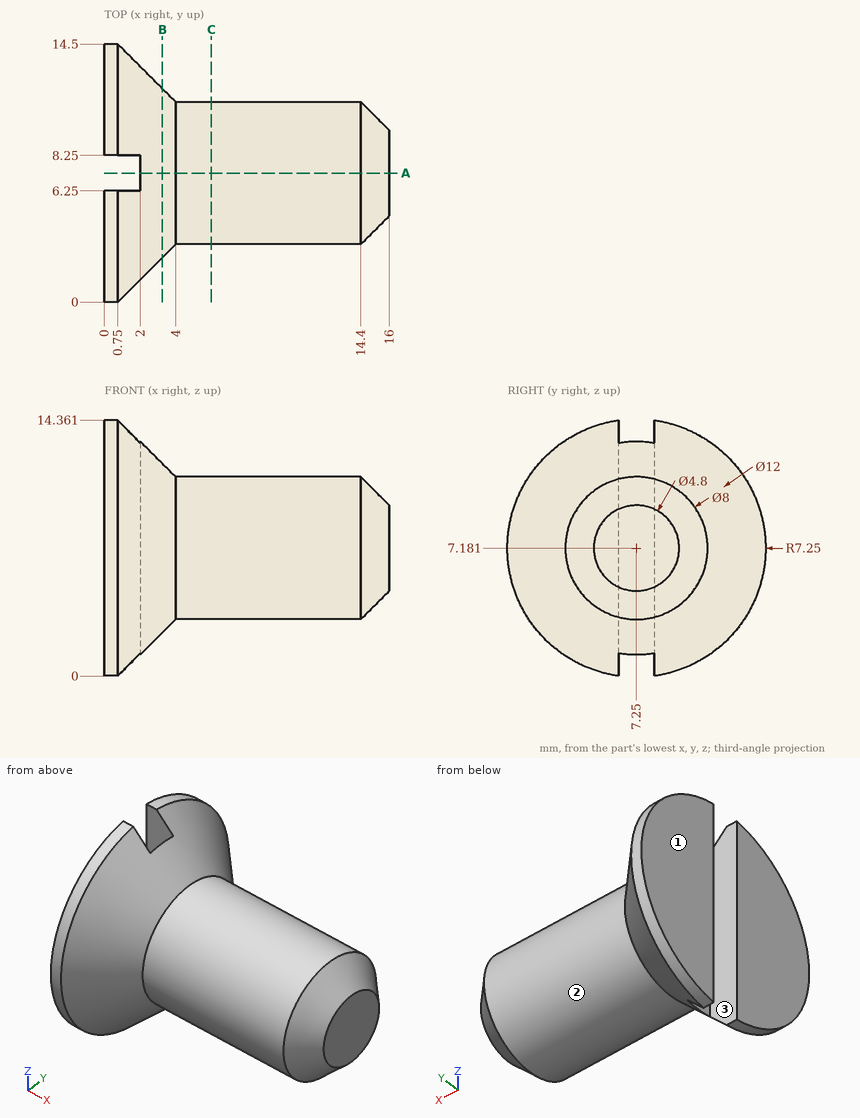
Here's the drawing with two shaded views (mm, measured from the low corner). I have some questions. A direction names the side the tool comes from. Give positions to 0.01 mm unless a question says otherwise; leave off trailing zeros. Write each loop counter-clockwise with the first axis right and the second up, starting at its lowest first coordinate (ties: lowest second). Pieces come first, ordered by that corner, then holes. Notation, with made-up numbers: (76, 12) -> (117, 12) arc R14 cw to (117, 28) -> close; hole circle Ø4 at (85.25, 53.5). An arc over 180 degrees is marked (long way). Answer as a JSON object with one key per item and string values. Group by question number.
Item 1: Suppose I cut it at C-C (x = 6). Please give me the cut outline in (y, z).
Item 2: Suppose I cut it at A-A (y = 7.25). Please give me the cut outline in (x, z), plus the area to 3 significant figures.
Item 3: For the marked faces 1, 2 and 3, which set-ups out of +Z, -Z, +X, -X, +Y, -Y let a thin tool reach every point of the face, with its end or its side?
Item 4: I'm going to push flat-ended pins straight in: P1, Ø8, axis at y = 8.5, z = 1.5, coming from the -X side; P2, Ø8, axis at x = 5.5, z = 4.5, coming from the -Y side; P3, Ø1.6, axis at x = 1, z = 6, coming from the -Y side; P4, Ø1, axis at x = 13, y = 1.5, coming from the +Z side. Where does each tip first touch, or does it pass through?
Item 5: Suppose I cut it at B-B (x = 3.25). Please give me the cut outline in (y, z).
Item 6: Please list where these lines run through material, in increasing order: line 1 (Z direction, x = 1, y = 12) (1 decimal); line 2 (X direction, y = 3.5, z = 4); line 3 (Z direction, x = 7.25, y = 9) (1 decimal). Write a range as [from, to].
Findings:
{
 "1": {"outline": "circle Ø8 at (7.25, 7.18)"},
 "2": {"outline": "(2, 1.18) -> (4, 3.18) -> (14.4, 3.18) -> (16, 4.78) -> (16, 9.58) -> (14.4, 11.18) -> (4, 11.18) -> (2, 13.18) -> close", "area": "113 mm²"},
 "3": {"face 1": "+Z, -Z, -X, +Y, -Y", "face 2": "+X", "face 3": "+Z, -Z, -X"},
 "4": {"P1": "stops at x = 0", "P2": "stops at y = 1.1", "P3": "stops at y = 0.01", "P4": "passes through"},
 "5": {"outline": "circle Ø9.5 at (7.25, 7.18)"},
 "6": {"line 1": "z = [2, 12.3]", "line 2": "x = [0, 3.08]", "line 3": "z = [3.6, 10.8]"}
}
